The figure shows three views and two pictorial views of one solid part (mm, origin at its lowest corner). Answer the questions. A direction names the side the tool comes from. Coordinates: 2 decimals unless noted, no trailing zeros. Order: outer loops, then holes, each group sorted by start corner. A loop starts at its lowest first (then second) coordinate and runs counter-clockwise, first axis right, second up. Notation, with made-up numbers: (-27, -3.5) -> (-9, -3.5) arc R24 cw to (-9, 6.5) -> close; hole circle Ø2 at (-31.5, 56.5). An arc over 180 degrees is marked (long way). Return JSON: item names as keys, results as strings.
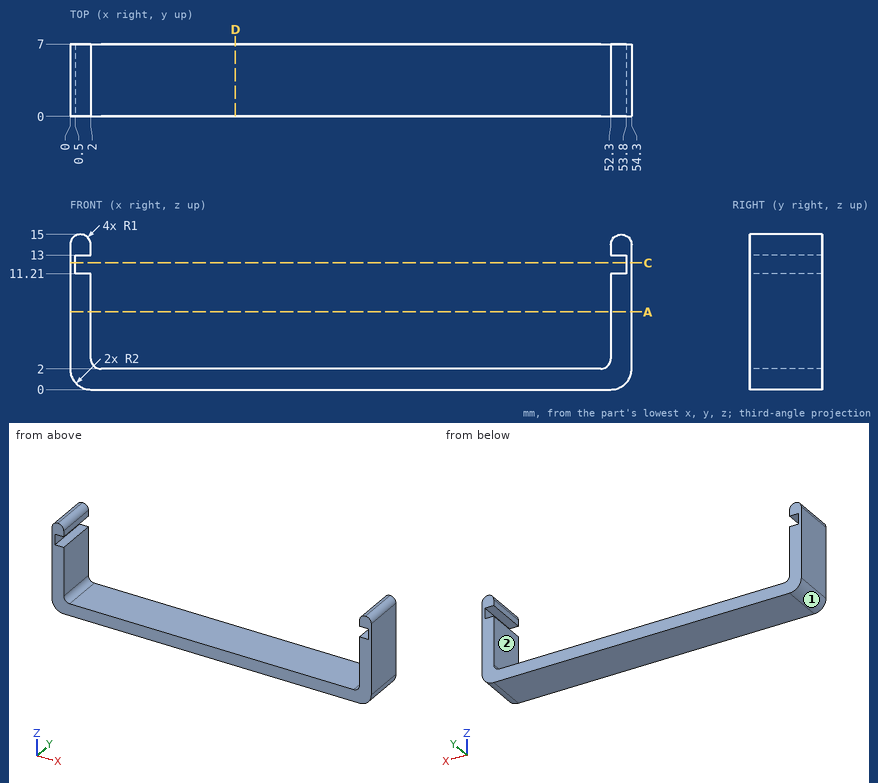
Item 1: Which of the six approach directions +Z, -Z, +X, -X, +Y, -Y give full straight-line access (tool end or side, diameter ignored) to the marked faces 1 and 2?
Answer list:
{"face 1": "-Z, -X, +Y, -Y", "face 2": "+Z, +Y, -Y"}
Item 2: Flat-ended cylindrical pins translate along their axes: pin 1 (4 mm diameter, centred on y = 6, z = 12.5, fed in from -X); pin 2 (1.5 mm diameter, centred on x = 31.5, y = 5.5, fed in from +Z); pin 3 (1.6 mm diameter, centred on x = 53.5, y = 3.5, fed in from -Z). Find the tip coordinate at first contact, or state that the pin passes through.
Answer list:
{"pin 1": "x = 0", "pin 2": "z = 2", "pin 3": "z = 0.04"}
Item 3: Find the intervals of material crossed by probe 1 along X at (y, z) = (6.75, 12); probe 2 along X at (y, z) = (2.75, 10.5); probe 3 along Z at (x, y) = (4, 5.75), in increasing order.
Answer list:
{"probe 1": "0 to 0.5, 53.8 to 54.3", "probe 2": "0 to 2, 52.3 to 54.3", "probe 3": "0 to 2"}
Item 4: The part is cut by section D-D on x = 16. Determine the outline of the cut face in (y, z), plus the area to 3 significant figures.
Answer list:
{"outline": "(0, 0) -> (7, 0) -> (7, 2) -> (0, 2) -> close", "area": "14.0 mm2"}
Item 5: The part is cut by section C-C on z = 12.25. Determine the outline of the cut face in (x, y).
Answer list:
{"outline": "(0, 0) -> (0.5, 0) -> (0.5, 7) -> (0, 7) -> close; (53.8, 0) -> (54.3, 0) -> (54.3, 7) -> (53.8, 7) -> close"}
Item 6: The part is cut by section A-A on z = 7.5. Determine the outline of the cut face in (x, y), plus the area to 3 significant figures.
Answer list:
{"outline": "(0, 0) -> (2, 0) -> (2, 7) -> (0, 7) -> close; (52.3, 0) -> (54.3, 0) -> (54.3, 7) -> (52.3, 7) -> close", "area": "28.0 mm2"}
